from build123d import *

# Parameters (mm, degrees)
SKETCH1_R           = 8.128
SKETCH1_R_2         = 4.191
BOSS_EXTRUDE1_DEPTH = 26.416
CUT_EXTRUDE1_REACH  = 60.42
SKETCH2_W           = 41.148
SKETCH2_H           = 20.32
CUT_EXTRUDE2_REACH  = 46.196
SKETCH3_R           = 4.125


with BuildPart() as part:
    # Sketch1 → Boss-Extrude1 (new body)
    with BuildSketch(Plane(origin=(0, 0, 0), x_dir=(1, 0, 0), z_dir=(0, 1, 0))):
        with BuildLine():
            Line((-58.42, 0), (0, 0))
            Line((0, 0), (0, 36.068))
            ThreePointArc((0, 36.068), (-12.241042079, 29.057488688), (-12.09332403, 43.163110242))
            Line((-12.09332403, 43.163110242), (-58.42, 17.272))
            Line((-58.42, 17.272), (-58.42, 0))
        make_face()
        with Locations((-8.128, 36.068)):
            Circle(SKETCH1_R)
        with Locations(Location((-8.128, 36.068, 0), (0, 0, 270))):  # turned: the seam where the file's is
            Circle(SKETCH1_R_2, mode=Mode.SUBTRACT)
    extrude(amount=-BOSS_EXTRUDE1_DEPTH)

    # Sketch2 → Cut-Extrude1 (cut, up to next)
    with BuildSketch(Plane(origin=(0, 0, 0), x_dir=(0, 0, -1), z_dir=(1, 0, 0)), mode=Mode.PRIVATE) as cut_extrude1_sk1:
        with Locations((23.622, -13.208)):
            Rectangle(SKETCH2_W, SKETCH2_H)
    cut_extrude1_tool1 = extrude(cut_extrude1_sk1.sketch, amount=-CUT_EXTRUDE1_REACH, mode=Mode.PRIVATE) & part.part
    add(cut_extrude1_tool1.solids().sort_by_distance((0, -13.208, -23.622))[0], mode=Mode.SUBTRACT)

    # Sketch3 → Cut-Extrude2 (cut, up to next)
    with BuildSketch(Plane.XY, mode=Mode.PRIVATE) as cut_extrude2_sk1:
        with Locations((-46.42, -13.208)):
            Circle(SKETCH3_R)
    cut_extrude2_tool1 = extrude(cut_extrude2_sk1.sketch, amount=-CUT_EXTRUDE2_REACH, mode=Mode.PRIVATE) & part.part
    add(cut_extrude2_tool1.solids().sort_by_distance((-46.42, -13.208, 0))[0], mode=Mode.SUBTRACT)
    # Sketch3 → Cut-Extrude2 (cut, up to next)
    with BuildSketch(Plane.XY, mode=Mode.PRIVATE) as cut_extrude2_sk2:
        with BuildLine():
            Line((0, -13.208), (0, -8.708))
            Line((0, -8.708), (-10, -8.708))
            ThreePointArc((-10, -8.708), (-14.5, -13.208), (-10, -17.708))
            Line((-10, -17.708), (0, -17.708))
            Line((0, -17.708), (0, -13.208))
        make_face()
    cut_extrude2_tool2 = extrude(cut_extrude2_sk2.sketch, amount=-CUT_EXTRUDE2_REACH, mode=Mode.PRIVATE) & part.part
    add(cut_extrude2_tool2.solids().sort_by_distance((-6.804413, -13.208, 0))[0], mode=Mode.SUBTRACT)


solid = part.part
Work out the finished part from the listing and answer in its coordinate system (mm). A direction names the side the tool comes from. Coordinates: 2 decimals unless noted, no trailing zeros. Loops run counter-clockwise (first coordinate to the right, second up) from the corner with the lowest first, then second, coordinate; pieces in that order, holes last. Notation, with made-up numbers: (74.25, 34.25) -> (111.25, 34.25) arc R28 ccw to (111.25, 61.25) -> close; hole circle Ø6 at (58, 82). An arc over 180 degrees is marked (long way). Answer as CSV lines item,"result".
1) The part is cut by section D-D (z = -38). Give the vertices of the cut face in (x, y).
A:
outline,"(-21.33, -26.42) -> (-11.85, -26.42) -> (-11.85, -23.37) -> (-21.33, -23.37) -> close; (-21.33, -3.05) -> (-11.85, -3.05) -> (-11.85, 0) -> (-21.33, 0) -> close; (-4.41, -26.42) -> (-0.23, -26.42) -> (-0.23, -23.37) -> (-4.41, -23.37) -> close; (-4.41, -3.05) -> (-0.23, -3.05) -> (-0.23, 0) -> (-4.41, 0) -> close"
2) The part is cut by section A-A (z = -24). Give the vertices of the cut face in (x, y), and give its area (3 significant figures).
A:
outline,"(-46.38, -26.42) -> (0, -26.42) -> (0, -23.37) -> (-46.38, -23.37) -> close; (-46.38, -3.05) -> (0, -3.05) -> (0, 0) -> (-46.38, 0) -> close"
area,"283 mm²"
3) The part is cut by section C-C (x = -7.5). Give the vertices of the cut face in (y, z), and give its area (3 significant figures).
A:
outline,"(-26.42, -44.17) -> (-23.37, -44.17) -> (-23.37, -40.21) -> (-26.42, -40.21) -> close; (-26.42, -31.92) -> (-23.37, -31.92) -> (-23.37, -3.05) -> (-17.71, -3.05) -> (-17.71, 0) -> (-26.42, 0) -> close; (-8.71, -3.05) -> (-3.05, -3.05) -> (-3.05, -31.92) -> (0, -31.92) -> (0, 0) -> (-8.71, 0) -> close; (-3.05, -44.17) -> (0, -44.17) -> (0, -40.21) -> (-3.05, -40.21) -> close"
area,"253 mm²"
4) For a pull along Y with two mould halves and no side action, classify faces 4 (the face through (-14.5, -13.1, -1.5)), 5 (the face through (-34.93, -1.5, -30.4)), 6 (the face through (-23, 0, -17)) as released by +Y, released by -Y, zero draft, split by the parting line, or undercut.
A:
face 4,"undercut"
face 5,"zero draft"
face 6,"released by +Y"
5) The part is cut by section B-B (y = -15.5). Give the vertices of the cut face in (x, z), and give its area (3 significant figures).
A:
outline,"(-58.42, -3.05) -> (-49.85, -3.05) -> (-49.85, 0) -> (-58.42, 0) -> close; (-42.99, -3.05) -> (-13.87, -3.05) -> (-13.87, 0) -> (-42.99, 0) -> close"
area,"115 mm²"
6) For faces 1 (the face through (-5, -17.708, -2)), 2 (the face through (-3.913, -1.503, -43.018)), 3 (the face through (-22, -3.048, -19)), determine the directions among +Z, -Z, +X, -X, +Y, -Y from which every point of the face is accessible in a straight line to the end or side of a thin tool.
A:
face 1,"+Z, -Z, +X"
face 2,"-Z, +Y, -Y"
face 3,"-Z, +X, -X"
7) Straight lines are drawn through the part: probe 1 along Y at (x, z) = (-12.5, -5); probe 2 along Z at (x, y) = (-42, -9.25); probe 3 along Y at (x, z) = (-46, -2). For each, find the intervals that lie inside material, in ascending order.
A:
probe 1,"y = -26.42 to -23.37, -3.05 to 0"
probe 2,"z = -3.05 to 0"
probe 3,"y = -26.42 to -17.31, -9.1 to 0"
8) Flat-ended cylindrical pins translate along their axes: pin 1 (13 mm diameter, centred on x = -46.42, y = -13.208, fed in from -Z); pin 2 (6.5 mm diameter, centred on x = -8.128, z = -36.068, fed in from -Y). Find the tip coordinate at first contact, or state that the pin passes through.
A:
pin 1,"stops at z = -3.05"
pin 2,"passes through"
